The drawing under review shows one solid part. Ordinate dimensions are in mm from its lowest x, y, z. Round coordinates to 2 decimals unless told otherwise and drop trailing zeros. Loops run counter-clockwise (first coordinate to the right, second up) from the corner with the lowest first, then second, coordinate; pieces in that order, holes last. Notation, with made-up numbers: (-3, -3.5) - (29, -3.5) arc R10 ccw to (29, 14.5) - close; hole circle Ø2 at (-33.75, 38). An arc over 180 degrees is marked (long way). Answer as CSV lines item,"result".
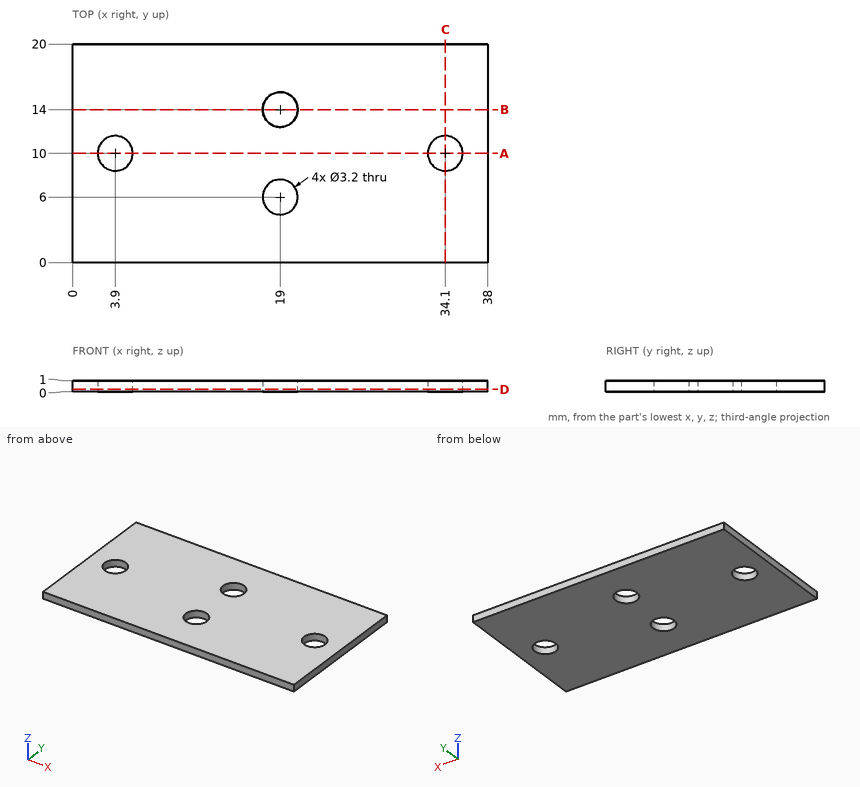
1. Wall thickness on probe 1 along Y at (x, z) = (19, 0.75); probe 2 along Y at (x, z) = (3.9, 0.65); probe 3 along X at (y, z) = (9.5, 0.1): over which ranges is each line inside the solid? List them lowest first.
Numbers:
probe 1,"y = 0 to 4.4, 7.6 to 12.4, 15.6 to 20"
probe 2,"y = 0 to 8.4, 11.6 to 20"
probe 3,"x = 0 to 2.38, 5.42 to 32.58, 35.62 to 38"
2. Clearance check with a flat-ended pin moving along its axis: pin 1 (1.9 mm diameter, centred on x = 19, y = 6, fed in from +Z). State where the tip first meets the part, or that it passes through.
Numbers:
pin 1,"passes through"
3. Take a section at A-A (y = 10). State the section outline as (x, z) points, plus the area to 3 significant figures.
Numbers:
outline,"(0, 0) - (2.3, 0) - (2.3, 1) - (0, 1) - close; (5.5, 0) - (32.5, 0) - (32.5, 1) - (5.5, 1) - close; (35.7, 0) - (38, 0) - (38, 1) - (35.7, 1) - close"
area,"31.6 mm²"
4. Take a section at C-C (x = 34.1). State the section outline as (y, z) points.
Numbers:
outline,"(0, 0) - (8.4, 0) - (8.4, 1) - (0, 1) - close; (11.6, 0) - (20, 0) - (20, 1) - (11.6, 1) - close"
5. Take a section at D-D (z = 0.2). State the section outline as (x, y) points.
Numbers:
outline,"(0, 0) - (38, 0) - (38, 20) - (0, 20) - close; hole circle Ø3.2 at (3.9, 10); hole circle Ø3.2 at (19, 6); hole circle Ø3.2 at (19, 14); hole circle Ø3.2 at (34.1, 10)"
6. Take a section at B-B (y = 14). State the section outline as (x, z) points, plus the area to 3 significant figures.
Numbers:
outline,"(0, 0) - (17.4, 0) - (17.4, 1) - (0, 1) - close; (20.6, 0) - (38, 0) - (38, 1) - (20.6, 1) - close"
area,"34.8 mm²"
